Source: CAD feature listing. Evaluate the final solid. Frame: model axes, mm. Face numbers are marked on the shaded views. A direction names the side the tool comes from. Coordinates: 2 decimals unless noted, no trailing zeros. Write each loop counter-clockwise with the first axis right and the second up, starting at its lowest first coordinate (ties: lowest second). Pieces come first, ordered by that corner, then holes. Notation, with made-up numbers: M 61.25,14 L 94.25,14 A10 ccw 94.25,19 Z; hole C 35,29.5 d2. An arc over 180 degrees is marked long. Answer as CSV lines item,"result". Start each with the question number.
1. Section B-B on z = -26. Return the cut outline in (x, y).
2. Line query: probe 1 along Y at (x, z) = (-93.65, -37.5); probe 2 along X at (y, z) = (70.5, -42.5); probe 3 along X at (y, z) = (34, -36.5). Output: solid intervals per line, ascending. Write a range as [from, to].
3. Section C-C on z = -37.5. Count the separate pieces of the cut face and the enclosed holes in it, plus the area to 3 significant figures.
4. Mould query, pull axis Z, two halves, no side actions, for the marked faces 1, 2, 3 and 4. Classes: pulls with the +Z half, pulls with the -Z half, needs draft (parallel to the pull), parting line crosses it, or undercut.
5. Reachability of the marked faces 5, 6 and 7 from +Z, -Z, +X, -X, +Y, -Y: full face, straight path, thin tool, end or side. Return the list, or none.
6. Section A-A on x = 18.5. Return the cut outline in (y, z).
7. Contact query for flat-ended pins moving along their axis: pin 1 Ø1 at (x, y) = (26, 87.5) entering from -Z; pin 2 Ø1 at (y, z) = (47.5, 2) entering from -X; pin 3 Ø1 at (x, y) = (26, 54) entering from +Z. Output: stop coordinate, or through.
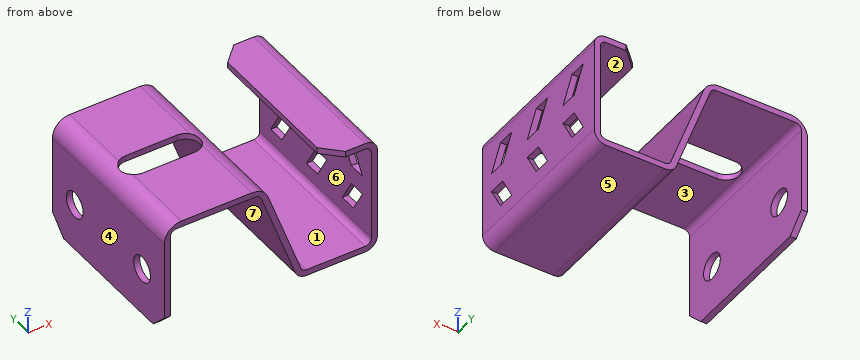
```python
from build123d import *

# Parameters (mm, degrees)
BOSS_EXTRUDE2_DEPTH = 100
CHAMFER1_SIZE       = 10
SKETCH2_R           = 7.5
CUT_EXTRUDE1_DEPTH  = 3.5
CUT_EXTRUDE2_DEPTH  = 3.5
CUT_EXTRUDE3_DEPTH  = 10
FILLET1_R           = 10


with BuildPart() as part:
    # Sketch1 → Boss-Extrude2 (new body)
    with BuildSketch(Plane(origin=(0, 0, 0), x_dir=(1, 0, 0), z_dir=(0, 1, 0))):
        with BuildLine():
            Line((0, 0), (21.5, 0))
            ThreePointArc((21.5, 0), (23.974873734, 1.025126266), (25, 3.5))
            Line((25, 3.5), (25, 56.5))
            ThreePointArc((25, 56.5), (23.974873734, 58.974873734), (21.5, 60))
            Line((21.5, 60), (-12.549273616, 60))
            ThreePointArc((-12.549273616, 60), (-14.556791143, 59.367032155), (-15.838197789, 57.697070502))
            Line((-15.838197789, 57.697070502), (-37.20218429, -1))
            Line((-37.20218429, -1), (-95, -1))
            Line((-95, -1), (-95, 65))
            Line((-95, 65), (-91.5, 65))
            Line((-91.5, 65), (-91.5, 6))
            ThreePointArc((-91.5, 6), (-90.474873734, 3.525126266), (-88, 2.5))
            Line((-88, 2.5), (-42.103637058, 2.5))
            ThreePointArc((-42.103637058, 2.5), (-40.09611953, 3.132967845), (-38.814712885, 4.802929498))
            Line((-38.814712885, 4.802929498), (-19.127121962, 58.894141003))
            ThreePointArc((-19.127121962, 58.894141003), (-16.564308671, 62.23406431), (-12.549273616, 63.5))
            Line((-12.549273616, 63.5), (21.5, 63.5))
            ThreePointArc((21.5, 63.5), (26.449747468, 61.449747468), (28.5, 56.5))
            Line((28.5, 56.5), (28.5, 3.5))
            ThreePointArc((28.5, 3.5), (26.449747468, -1.449747468), (21.5, -3.5))
            Line((21.5, -3.5), (0, -3.5))
            Line((0, -3.5), (0, 0))
        make_face()
    extrude(amount=BOSS_EXTRUDE2_DEPTH)

    # Chamfer1
    chamfer1_edges = [part.edges().sort_by_distance(p)[0] for p in [
        (-93.25, 0, -65),
        (0, 0, 1.75),
        (0, 100, 1.75),
        (-93.25, 100, -65),
    ]]
    chamfer(chamfer1_edges, length=CHAMFER1_SIZE)

    # Sketch2 → Cut-Extrude1 (cut)
    with BuildSketch(Plane.ZY.offset(95)):
        with Locations((-37.5, 19.9)):
            Circle(SKETCH2_R)
        with Locations((-37.5, 80.1)):
            Circle(SKETCH2_R)
    extrude(amount=-CUT_EXTRUDE1_DEPTH, mode=Mode.SUBTRACT)

    # Sketch3 → Cut-Extrude2 (cut)
    with BuildSketch(Plane(origin=(0, 0, -2.5), x_dir=(-1, 0, 0), z_dir=(0, 0, -1))):
        with BuildLine():
            Line((50.069082037, 58), (80.069082037, 58))
            ThreePointArc((80.069082037, 58), (88.069082037, 50), (80.069082037, 42))
            Line((80.069082037, 42), (50.069082037, 42))
            ThreePointArc((50.069082037, 42), (42.069082037, 50), (50.069082037, 58))
        make_face()
    extrude(amount=-CUT_EXTRUDE2_DEPTH, mode=Mode.SUBTRACT)

    # Sketch4 → Cut-Extrude3 (cut)
    with BuildSketch(Plane(origin=(28.5, 0, 0), x_dir=(0, 0, -1), z_dir=(1, 0, 0))):
        Polygon((48.5, 26.082903769), (48.5, 16.082903769), (34.5, 8), (34.5, 18), align=None)
        Polygon((23.5, 18), (23.5, 8), (9.5, 16.082903769), (9.5, 26.082903769), align=None)
        Polygon((48.5, 58.082903769), (48.5, 48.082903769), (34.5, 40), (34.5, 50), align=None)
        Polygon((23.5, 50), (23.5, 40), (9.5, 48.082903769), (9.5, 58.082903769), align=None)
        Polygon((48.5, 90.082903769), (48.5, 80.082903769), (34.5, 72), (34.5, 82), align=None)
        Polygon((23.5, 82), (23.5, 72), (9.5, 80.082903769), (9.5, 90.082903769), align=None)
    extrude(amount=-CUT_EXTRUDE3_DEPTH, mode=Mode.SUBTRACT)

    # Fillet1
    # the kernel refuses this fillet: 10 mm, written as the material it takes off along each edge
    with BuildSketch(Plane(origin=(-37.20218429, -17.505188455, 1), x_dir=(0.3420201433256651, 0, -0.9396926207859098), z_dir=(0, 1, 0))) as fillet1_piece_1:
        with BuildLine():
            CenterArc((FILLET1_R * 0.70020753821, FILLET1_R), FILLET1_R, 200, 70)
            Line((-FILLET1_R * 0.239485082576, FILLET1_R * 0.657979856674), (0, 0))
            Line((0, 0), (FILLET1_R * 0.70020753821, 0))
        make_face()
    extrude(amount=135.01037691, mode=Mode.SUBTRACT)
    with BuildSketch(Plane(origin=(-95, -25, 1), x_dir=(1, 0, 0), z_dir=(0, 1, 0))) as fillet1_piece_2:
        with BuildLine():
            CenterArc((FILLET1_R, FILLET1_R), FILLET1_R, 180, 90)
            Line((0, FILLET1_R), (0, 0))
            Line((0, 0), (FILLET1_R, 0))
        make_face()
    extrude(amount=150, mode=Mode.SUBTRACT)


solid = part.part
```
Values:
1,outline,"M -95,0 L -91.5,0 L -91.5,100 L -95,100 Z; M -31.1,0 L -27.37,0 L -27.37,100 L -31.1,100 Z; M 25,0 L 28.5,0 L 28.5,100 L 25,100 Z"
2,probe 1,"[0, 12.4], [27.4, 72.6], [87.6, 100]"
2,probe 2,"[-95, -91.5], [-25.09, -21.37], [25, 28.5]"
2,probe 3,"[-95, -91.5], [-27.28, -23.55], [25, 28.5]"
3,separate pieces,"8"
3,enclosed holes,"0"
3,area,"862 mm²"
4,face 1,"undercut"
4,face 2,"undercut"
4,face 3,"pulls with the -Z half"
4,face 4,"needs draft"
5,face 5,"-Z, +X, +Y, -Y"
5,face 6,"+Y, -Y"
5,face 7,"-Z, +Y, -Y"
6,outline,"M 0,-63.5 L 100,-63.5 L 100,-60 L 0,-60 Z; M 0,0 L 100,0 L 100,3.5 L 0,3.5 Z"
7,pin 1,"z = -62.24"
7,pin 2,"x = 0"
7,pin 3,"z = 2.24"
